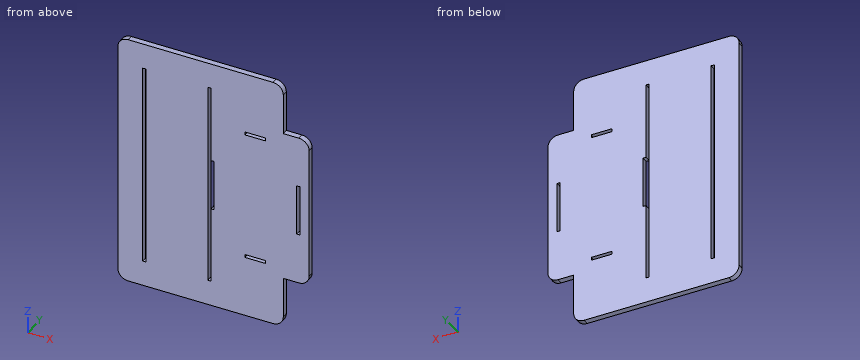
Autodesk Inventor part; units mm, degrees
ref_plane "YZ Plane" through (0, 0, 0) normal (1, 0, 0) x (0, 1, 0)
ref_plane "XZ Plane" through (0, 0, 0) normal (0, 1, 0) x (-1, 0, 0)
ref_plane "XY Plane" through (0, 0, 0) normal (0, 0, 1) x (1, 0, 0)
sketch "Sketch1" plane through (0, 0, 0) normal (0, 1, 0) x (-1, 0, 0)
  line L0 (204.2348, 103.8462) -> (44.2348, 103.8462)
  line L1 (44.2348, 103.8462) -> (44.2348, -146.1538) construction
  line L2 (44.2348, -146.1538) -> (204.2348, -146.1538)
  line L3 (204.2348, -146.1538) -> (204.2348, 103.8462)
  line L4 (124.2348, 103.8462) -> (124.2348, -146.1538) construction
  line L5 (204.2348, -21.1538) -> (44.2348, -21.1538) construction
  line L6 (180.2348, 78.8462) -> (177.2348, 78.8462)
  line L7 (177.2348, 78.8462) -> (177.2348, -121.1538)
  line L8 (177.2348, -121.1538) -> (180.2348, -121.1538)
  line L9 (180.2348, -121.1538) -> (180.2348, 78.8462)
  line L10 (117.2348, 78.8462) -> (114.2348, 78.8462)
  line L11 (114.2348, 78.8462) -> (114.2348, -121.1538)
  line L12 (114.2348, -121.1538) -> (117.2348, -121.1538)
  line L13 (117.2348, -121.1538) -> (117.2348, 78.8462)
  line L14 (44.2348, -146.1538) -> (44.2348, -96.1538)
  line L15 (44.2348, 103.8462) -> (44.2348, 53.8462)
  line L16 (44.2348, -96.1538) -> (19.2348, -96.1538)
  line L17 (19.2348, -96.1538) -> (19.2348, 53.8462)
  line L18 (19.2348, 53.8462) -> (44.2348, 53.8462)
  point P0 (0, 0)
  dimension "d0" = 160
  dimension "d1" = 250
  dimension "d2" = 3
  dimension "d3" = 3
  dimension "d4" = 200
  dimension "d7" = 60
  dimension "d9" = 150
  dimension "d10" = 25
  dimension "d27" = 70
extrude "Extrusion2" add sketch "Sketch1" along normal blind 5.6
fillet "Fillet2" radius 10 6 edges at (-19.2348, 2.8, 53.8462) (-19.2348, 2.8, -96.1538) (-44.2348, 2.8, 103.8462) (-44.2348, 2.8, -146.1538) (-204.2348, 2.8, -146.1538) (-204.2348, 2.8, 103.8462)
sketch "Sketch3" plane through (0, 5.6, 0) normal (0, 1, 0) x (1, 0, 0)
  line L0 (-114.2348, 121.1538) -> (-114.2348, -78.8462)
  line L1 (-114.2348, 21.1538) -> (-19.2348, 21.1538) construction
  line L2 (-19.2348, -43.8462) -> (-19.2348, 86.1538)
  line L3 (-114.2348, 46.1538) -> (-111.2348, 46.1538)
  line L4 (-111.2348, 46.1538) -> (-111.2348, -3.8462)
  line L5 (-111.2348, -3.8462) -> (-114.2348, -3.8462)
  line L6 (-81.2348, 86.1538) -> (-81.2348, 83.1538)
  line L7 (-81.2348, 83.1538) -> (-61.2348, 83.1538)
  line L8 (-61.2348, 83.1538) -> (-61.2348, 86.1538)
  line L9 (-61.2348, 86.1538) -> (-81.2348, 86.1538)
  line L10 (-61.2348, -43.8462) -> (-81.2348, -43.8462)
  line L11 (-81.2348, -43.8462) -> (-81.2348, -40.8462)
  line L12 (-81.2348, -40.8462) -> (-61.2348, -40.8462)
  line L13 (-61.2348, -40.8462) -> (-61.2348, -43.8462)
  line L14 (-31.2348, 46.1538) -> (-31.2348, -3.8462)
  line L15 (-31.2348, -3.8462) -> (-28.2348, -3.8462)
  line L16 (-28.2348, -3.8462) -> (-28.2348, 46.1538)
  line L17 (-28.2348, 46.1538) -> (-31.2348, 46.1538)
  line L18 (-111.2348, 13.6812) -> (-31.2348, 13.6812) construction
  line L19 (-71.2348, 13.6812) -> (-71.2348, 32.3126) construction
  point P0 (0, 0)
  point P1 (-81.2348, -42.3462)
  dimension "d28" = 3
  dimension "d29" = 50
  dimension "d30" = 3
  dimension "d31" = 3
  dimension "d32" = 20
  dimension "d34" = 3
  dimension "d38" = 80
extrude "Extrusion4" cut sketch "Sketch3" against normal blind 10
equation "\"d0\" = BaseDepth"
equation "\"d1\" = BaseLength"
equation "\"d2\" = Width"
equation "\"d3\" = Width"
equation "\"d4\" = SlotLength"
equation "\"d28\" = Width"
equation "\"d30\" = Width"
equation "\"d31\" = Width"
equation "\"d34\" = Width"
equation "\"BaseDepth\" = 160"
equation "\"BaseLength\" = 250"
equation "\"Width\" = 3"
equation "\"SlotLength\" = 200"
properties part number "Base" material "ABS Plastic"
Read the model definition and answer for the solid it produces. Units are mm, in the model's axes. Coordinates: 2 decimals unless noted, no trailing zeros. Loops run counter-clockwise (first coordinate to the right, second up) from the corner with the lowest first, then second, coordinate; pieces in that order, holes last.
Q1. The part is cut by section D-D on x = -40. Write down the section's boundary in (y, z), and give its area (3 significant figures).
Q2. This flat-tipped pin is pushed along its axis until it touches: pin 1 Ø1.5 at (x, z) = (-138, -55.5) entering from -Y. Where does it stop, or does it pass through?
Q3. The part is cut by section B-B on x = -65. Write down the section's boundary in (y, z).
Q4. Consider probe 1 along X at (y, z) = (3.3, -38); probe 2 along Z at (x, y) = (-66.5, 3.6); probe 3 along X at (y, z) = (0.45, -63). Determine where each line is inside the solid, lowest interval first.
Q5. The part is cut by section A-A on z = -112.5. Write down the section's boundary in (x, y).
Q6. The part is cut by section C-C on y = 1. Give the number of separate pieces and of enclosed holes in the cut face, and give its area (3 significant figures).
Results below:
1. outline: (0, -96.15) - (5.6, -96.15) - (5.6, 53.85) - (0, 53.85) - close
1. area: 840 mm2
2. pin 1: stops at y = 0
3. outline: (0, -146.15) - (5.6, -146.15) - (5.6, -86.15) - (0, -86.15) - close; (0, -83.15) - (5.6, -83.15) - (5.6, 40.85) - (0, 40.85) - close; (0, 43.85) - (5.6, 43.85) - (5.6, 103.85) - (0, 103.85) - close
4. probe 1: x = -204.23 to -180.23, -177.23 to -117.23, -111.23 to -31.23, -28.23 to -19.23
4. probe 2: z = -146.15 to -86.15, -83.15 to 40.85, 43.85 to 103.85
4. probe 3: x = -204.23 to -180.23, -177.23 to -117.23, -114.23 to -19.23
5. outline: (-204.23, 0) - (-180.23, 0) - (-180.23, 5.6) - (-204.23, 5.6) - close; (-177.23, 0) - (-117.23, 0) - (-117.23, 5.6) - (-177.23, 5.6) - close; (-114.23, 0) - (-44.23, 0) - (-44.23, 5.6) - (-114.23, 5.6) - close
6. separate pieces: 1
6. enclosed holes: 5
6. area: 42,000 mm2
